For this review, take the finished solid that the model builds, in its own axes (mm). A direction names the side the tool comes from. Round coordinates to 2 decimals unless told otherwise and drop trailing zeros. Loops run counter-clockwise (first coordinate to the right, second up) from the corner with the lowest first, then second, coordinate; pieces in that order, holes last. Notation, with made-up numbers: M 71,55.25 L 129,55.25 A22 cw 129,84.25 Z; hole C 88,-39.5 d1. An arc over 180 degrees is marked long. Write item = value, one per line. Start each with the question number.
```python
from build123d import *

# Parameters (mm, degrees)
SKETCH3_W           = 22
SKETCH3_H           = 34.2
SKETCH3_W_2         = 12
SKETCH3_H_2         = 24.2
BOSS_EXTRUDE1_DEPTH = 16
SKETCH4_W           = 22
SKETCH4_H           = 10
BOSS_EXTRUDE2_DEPTH = 5
CUT_EXTRUDE6_DEPTH  = 3
SKETCH12_R          = 2.7
CUT_EXTRUDE7_DEPTH  = 3


with BuildPart() as part:
    # Sketch3 → Boss-Extrude1 (new body)
    with BuildSketch(Plane(origin=(0, 0, 0), x_dir=(1, 0, 0), z_dir=(0, 1, 0))):
        with Locations((6, 14.151918963)):
            Rectangle(SKETCH3_W, SKETCH3_H)
        with Locations((6, 14.151918963)):
            Rectangle(SKETCH3_W_2, SKETCH3_H_2, mode=Mode.SUBTRACT)
    extrude(amount=BOSS_EXTRUDE1_DEPTH)

    # Sketch4 → Boss-Extrude2 (add)
    with BuildSketch(Plane(origin=(0, 0, 0), x_dir=(1, 0, 0), z_dir=(0, 1, 0))):
        with Locations((6, 36.251918963)):
            Rectangle(SKETCH4_W, SKETCH4_H)
        with Locations((6, -7.948081037)):
            Rectangle(SKETCH4_W, SKETCH4_H)
    extrude(amount=BOSS_EXTRUDE2_DEPTH)

    # Sketch8 → Cut-Extrude6 (cut)
    with BuildSketch(Plane(origin=(0, 5, 0), x_dir=(1, 0, 0), z_dir=(0, 1, 0))):
        with BuildLine():
            Line((1, 36.251918963), (1, 41.251918963))
            Line((1, 41.251918963), (11, 41.251918963))
            Line((11, 41.251918963), (11, 36.251918963))
            ThreePointArc((11, 36.251918963), (9.535533906, 32.716385057), (6, 31.251918963))
            ThreePointArc((6, 31.251918963), (2.464466094, 32.716385057), (1, 36.251918963))
        make_face()
        with BuildLine():
            Line((1, -7.948081037), (1, -12.948081037))
            Line((1, -12.948081037), (11, -12.948081037))
            Line((11, -12.948081037), (11, -7.948081037))
            ThreePointArc((11, -7.948081037), (9.535533906, -4.412547131), (6, -2.948081037))
            ThreePointArc((6, -2.948081037), (2.464466094, -4.412547131), (1, -7.948081037))
        make_face()
    extrude(amount=-CUT_EXTRUDE6_DEPTH, mode=Mode.SUBTRACT)

    # Sketch12 → Cut-Extrude7 (cut)
    with BuildSketch(Plane.XZ):
        with Locations(Location((6, 7.948081037, 0), (0, 0, 270))):
            Circle(SKETCH12_R)
        with Locations(Location((6, -36.251918963, 0), (0, 0, 270))):
            Circle(SKETCH12_R)
    extrude(amount=-CUT_EXTRUDE7_DEPTH, mode=Mode.SUBTRACT)


solid = part.part
```
(1) For pin 1 Ø3 at (x, z) = (6, -36.25) entering from +Y; pin 2 Ø3 at (x, y) = (10, 9.5) entering from -Z; pin 3 Ø8 at (x, z) = (0, 8.5) entering from +Y; pin 4 Ø8 at (x, z) = (1.5, -34.5) entering from +Y, all flat-tipped, find the tip position at first contact; note any pin that passes through.
(2) Add section C-C on x = 5.5. Count the separate pieces of the cut face and the enclosed holes in it, and give its area (3 significant figures).
(3) Add section D-D on x = 9.25. Write out the cut boundary in (y, z), and give its area (3 significant figures).
(4) Add section A-A on y = 9.5. Write out the cut boundary in (x, z), and give its area (3 significant figures).
(5) Draft analysis for pull direction X (two halves, no side actions). For faces 1 (the flat face through (6, 8, -2.052)), 2 (the flat face through (14, 5, 8)), 3 (the flat face through (17, 6, -14)), 4 (the flat face through (-5, 6, -14)), state which applies: +X half, -X half, draft (parallel to the pull), parting line (faces both ways), or undercut.
(6) Add section B-B on z = -24.5. Write out the cut boundary in (x, y), and give its area (3 significant figures).
(7) Tool access review of faces 5 (the flat face through (4, 2, -39)), 6 (the flat face through (-2, 5, -36)), 7 (the flat face through (-2, 5, 8)): name each direction out of +Z, -Z, +X, -X, +Y, -Y from which nothing blocks a thin tool from reaching the whole face with its end or side.
(8) Wall thickness on L1, parallel to Z at x = 1, y = 8.5; L2, parallel to Z at x = 0.5, y = 4.75; L3, parallel to X at y = 8, z = -19.5: over which ranges is each line inside the solid? List them lowest first.
Answer sheet:
q1.pin_1 = through
q1.pin_2 = -31.25
q1.pin_3 = 5
q1.pin_4 = 16
q2.separate_pieces = 4
q2.enclosed_holes = 0
q2.area = 179 mm²
q3.outline = M 0,-41.25 L 2,-41.25 L 2,-32.45 L 5,-32.45 L 5,-31.25 L 16,-31.25 L 16,-26.25 L 0,-26.25 Z; M 0,-2.05 L 16,-2.05 L 16,2.95 L 5,2.95 L 5,4.15 L 2,4.15 L 2,12.95 L 0,12.95 Z
q3.area = 207 mm²
q4.outline = M -5,-31.25 L 17,-31.25 L 17,2.95 L -5,2.95 Z; hole M 0,-26.25 L 12,-26.25 L 12,-2.05 L 0,-2.05 Z
q4.area = 462 mm²
q5.face_1 = undercut
q5.face_2 = draft
q5.face_3 = +X half
q5.face_4 = -X half
q6.outline = M -5,0 L 0,0 L 0,16 L -5,16 Z; M 12,0 L 17,0 L 17,16 L 12,16 Z
q6.area = 160 mm²
q7.face_5 = -Z, +Y
q7.face_6 = -Z, +X, -X, +Y
q7.face_7 = +Z, +X, -X, +Y
q8.L1 = -31.25 to -26.25, -2.05 to 2.95
q8.L2 = -41.25 to -26.25, -2.05 to 12.95
q8.L3 = -5 to 0, 12 to 17
